Design review of the part built by this model. Coordinates are the model's own, in mm. A direction names the side the tool comes from. Coordinates: 2 decimals unless noted, no trailing zeros. Write each loop counter-clockwise with the first axis right and the second up, starting at its lowest first coordinate (ties: lowest second). Pieces come first, ordered by that corner, then holes. Notation, with made-up numbers: (86, 51) - (104, 51) arc R16 ccw to (104, 70) - close; hole circle Ø9 at (68.25, 7.5). An arc over 180 degrees is marked (long way). Answer as CSV lines item,"result". Start each with the question number.
Q1. For line 1 along Z through (x, y) = (10, -1); line 2 along Y through (x, z) = (150.75, 200); line 3 along Y through (x, z) = (151.4, 350), list the stretches that pass through material, from the lowest coordinate up. Write a range as [from, to].
Q2. Machinability: for faces 1 (the face through (150, -116, 197)), 2 (the face through (152, -104, 197)), which of the approach directions +Z, -Z, +X, -X, +Y, -Y give a long, thin tool a straight path to every point of the face, cutting with its end or side? Answer none if there is none.
Q3. We need section A-A (y = -56). Write out the cut boundary in (x, z), plus the area to 3 significant figures.
Q4. We need section C-C (z = 121). Write out the cut boundary in (x, y), plus the area to 3 significant figures.
Q5. Clearance check with flat-ended pins moving along their axes: pin 1 (2.5 mm diameter, centred on x = 10, z = 50, fed in from +Y); pin 2 (6.5 mm diameter, centred on x = 138, z = 50, fed in from -Y); pin 3 (2 mm diameter, centred on y = -1.5, z = 255, fed in from +X); pin 4 (5 mm diameter, centred on y = -14, z = 200, fed in from -X). State where each tip first meets the part, or that it passes through.
Q6. We need section B-B (x = 96.5). Write out the cut boundary in (y, z), plus the area to 3 significant figures.
from build123d import *

# Parameters (mm, degrees)
BOSS_EXTRUDE1_DEPTH = 400
SKETCH3_W           = 340
SKETCH3_H           = 79
CUT_EXTRUDE1_DEPTH  = 2
SKETCH4_W           = 108
SKETCH4_H           = 340
CUT_EXTRUDE2_DEPTH  = 2
SKETCH6_R           = 3.25
CUT_EXTRUDE3_DEPTH  = 2
SKETCH7_R           = 2
CUT_EXTRUDE4_DEPTH  = 2
SKETCH8_R           = 2
CUT_EXTRUDE5_DEPTH  = 2


with BuildPart() as part:
    # Sketch1 → Boss-Extrude1 (new body)
    with BuildSketch(Plane.XY):
        with BuildLine():
            Line((0, 0), (0, -2))
            Line((0, -2), (146, -2))
            ThreePointArc((146, -2), (148.828427125, -3.171572875), (150, -6))
            Line((150, -6), (150, -123))
            Line((150, -123), (152, -123))
            Line((152, -123), (152, -4))
            ThreePointArc((152, -4), (150.828427125, -1.171572875), (148, 0))
            Line((148, 0), (0, 0))
        make_face()
    extrude(amount=BOSS_EXTRUDE1_DEPTH)

    # Sketch3 → Cut-Extrude1 (cut)
    with BuildSketch(Plane(origin=(152, 0, 0), x_dir=(0, 0, -1), z_dir=(1, 0, 0))):
        with Locations((-190, -63.5)):
            Rectangle(SKETCH3_W, SKETCH3_H)
    extrude(amount=-CUT_EXTRUDE1_DEPTH, mode=Mode.SUBTRACT)

    # Sketch4 → Cut-Extrude2 (cut)
    with BuildSketch(Plane(origin=(0, 0, 0), x_dir=(1, 0, 0), z_dir=(0, 1, 0))):
        with Locations((74, -190)):
            Rectangle(SKETCH4_W, SKETCH4_H)
    extrude(amount=-CUT_EXTRUDE2_DEPTH, mode=Mode.SUBTRACT)

    # Sketch6 → Cut-Extrude3 (cut)
    with BuildSketch(Plane(origin=(152, 0, 0), x_dir=(0, 0, -1), z_dir=(1, 0, 0))):
        with Locations((-385, -14)):
            Circle(SKETCH6_R)
        with Locations((-385, -113)):
            Circle(SKETCH6_R)
    extrude(amount=-CUT_EXTRUDE3_DEPTH, mode=Mode.SUBTRACT)

    # Sketch7 → Cut-Extrude4 (cut)
    with BuildSketch(Plane(origin=(0, 0, 0), x_dir=(1, 0, 0), z_dir=(0, 1, 0))):
        with Locations(Location((10, -50, 0), (0, 0, 180))):
            Circle(SKETCH7_R)
        with Locations(Location((10, -200, 0), (0, 0, 180))):
            Circle(SKETCH7_R)
        with Locations(Location((10, -350, 0), (0, 0, 180))):
            Circle(SKETCH7_R)
        with Locations(Location((138, -50, 0), (0, 0, 180))):
            Circle(SKETCH7_R)
        with Locations(Location((138, -200, 0), (0, 0, 180))):
            Circle(SKETCH7_R)
        with Locations(Location((138, -350, 0), (0, 0, 180))):
            Circle(SKETCH7_R)
    extrude(amount=-CUT_EXTRUDE4_DEPTH, mode=Mode.SUBTRACT)

    # Sketch8 → Cut-Extrude5 (cut)
    with BuildSketch(Plane(origin=(152, 0, 0), x_dir=(0, 0, -1), z_dir=(1, 0, 0))):
        with Locations((-50, -113)):
            Circle(SKETCH8_R)
        with Locations((-200, -113)):
            Circle(SKETCH8_R)
        with Locations((-350, -113)):
            Circle(SKETCH8_R)
        with Locations(Location((-350, -14, 0), (0, 0, 180))):
            Circle(SKETCH8_R)
        with Locations(Location((-200, -14, 0), (0, 0, 180))):
            Circle(SKETCH8_R)
        with Locations(Location((-50, -14, 0), (0, 0, 180))):
            Circle(SKETCH8_R)
    extrude(amount=-CUT_EXTRUDE5_DEPTH, mode=Mode.SUBTRACT)


solid = part.part
Results list:
1,line 1,"z = [0, 48], [52, 198], [202, 348], [352, 400]"
1,line 2,"y = [-123, -115], [-111, -103], [-24, -16], [-12, -1.1]"
1,line 3,"y = [-123, -115], [-111, -103], [-24, -16], [-12, -1.89]"
2,face 1,"+Z, -Z, -X, -Y"
2,face 2,"+Z, -Z, +X, +Y, -Y"
3,outline,"(150, 0) - (152, 0) - (152, 20) - (150, 20) - close; (150, 360) - (152, 360) - (152, 400) - (150, 400) - close"
3,area,"120 mm2"
4,outline,"(0, -2) - (20, -2) - (20, 0) - (0, 0) - close; (128, -2) - (146, -2) arc R4 cw to (150, -6) - (150, -24) - (152, -24) - (152, -4) arc R4 ccw to (148, 0) - (128, 0) - close; (150, -123) - (152, -123) - (152, -103) - (150, -103) - close"
4,area,"172 mm2"
5,pin 1,"passes through"
5,pin 2,"stops at y = -2"
5,pin 3,"stops at x = 151.71"
5,pin 4,"stops at x = 150"
6,outline,"(-2, 0) - (0, 0) - (0, 20) - (-2, 20) - close; (-2, 360) - (0, 360) - (0, 400) - (-2, 400) - close"
6,area,"120 mm2"
